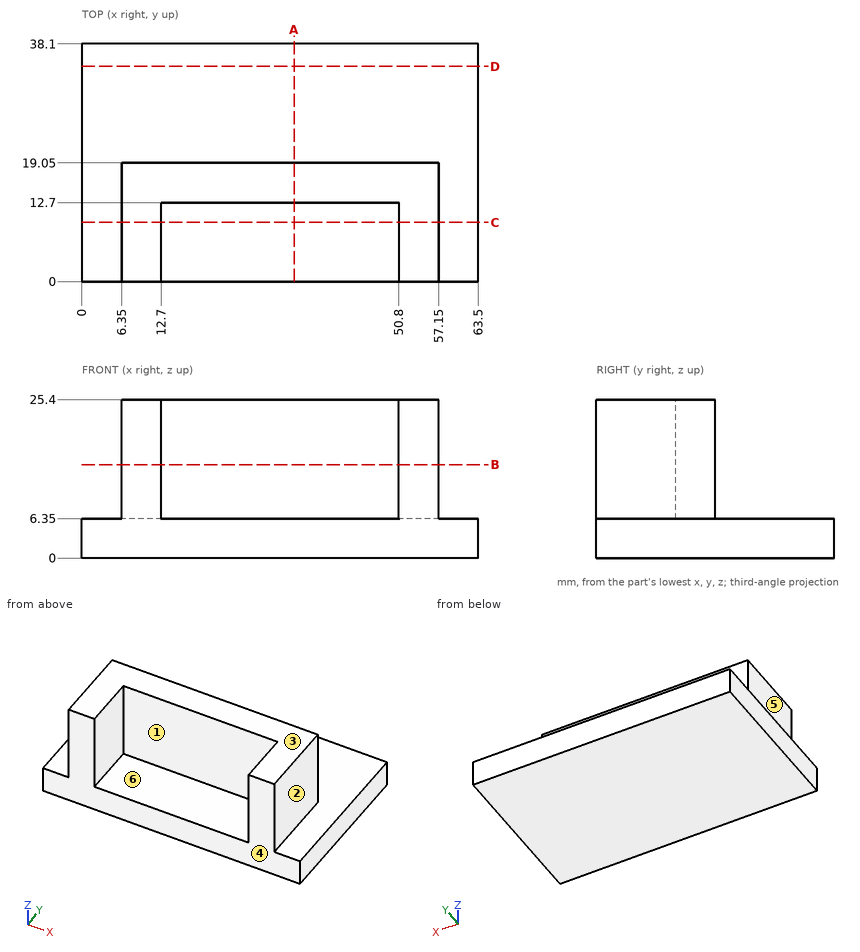
Print and shaded views of the part. All mm, measured from the part's lowest x, y and z. A direction names the side the tool comes from. Round coordinates to 2 decimals unless told otherwise and drop trailing zeros. Write each loop counter-clockwise with the first axis right and the second up, starting at its lowest first coordinate (ties: lowest second). Pieces come first, ordered by that corner, then holes.
Item 1: Cut at B-B, the plane z = 15. Give the cut face in (x, y).
Results:
outline: (6.35, 0) - (12.7, 0) - (12.7, 12.7) - (50.8, 12.7) - (50.8, 0) - (57.15, 0) - (57.15, 19.05) - (6.35, 19.05) - close
Item 2: Probe L1, parallel to Y at x = 51, z = 10.75; L2, parallel to Y at x = 15, z = 16; L3, parallel to X at y = 6.5, z = 20. List the from-to ranges inside material, lowest first.
Results:
L1: y = 0 to 19.05
L2: y = 12.7 to 19.05
L3: x = 6.35 to 12.7, 50.8 to 57.15
Item 3: Cut at C-C, the plane y = 9.5. Give the cut face in (x, z).
Results:
outline: (0, 0) - (63.5, 0) - (63.5, 6.35) - (57.15, 6.35) - (57.15, 25.4) - (50.8, 25.4) - (50.8, 6.35) - (12.7, 6.35) - (12.7, 25.4) - (6.35, 25.4) - (6.35, 6.35) - (0, 6.35) - close
Item 4: Cut at D-D, the plane y = 34.5. Give the cut face in (x, z), plus the area to 3 significant figures.
Results:
outline: (0, 0) - (63.5, 0) - (63.5, 6.35) - (0, 6.35) - close
area: 403 mm2
Item 5: Drop flat-ended pins along their axis: pin 1 Ø6 at (y, z) = (5.5, 10.5) entering from -X; pin 2 Ø5.5 at (y, z) = (14.5, 13.5) entering from +X; pin 3 Ø2 at (x, y) = (51, 22.5) entering from +Z. Give the stop position or say it passes through.
Results:
pin 1: stops at x = 6.35
pin 2: stops at x = 57.15
pin 3: stops at z = 6.35
Item 6: Which spindle directions (+Z, -Z, +X, -X, +Y, -Y) get a long thin tool onto all of the face, cutting with end or side? Do the marked faces 1, 2 and 3. Say none if no direction does.
Results:
face 1: +Z, -Y
face 2: +Z, +X, +Y, -Y
face 3: +Z, +X, -X, +Y, -Y
Item 7: Cut at A-A, the plane x = 34. Give the cut face in (y, z).
Results:
outline: (0, 0) - (38.1, 0) - (38.1, 6.35) - (19.05, 6.35) - (19.05, 25.4) - (12.7, 25.4) - (12.7, 6.35) - (0, 6.35) - close
Item 8: Two-plate mould, pull along X, no slides. Class the marked faces 4, 5 and 6: +X half, -X half, draft (parallel to the pull), parting line (faces both ways), or undercut.
Results:
face 4: draft
face 5: -X half
face 6: undercut
